from build123d import *

# Parameters (mm, degrees)
SKETCH2_W           = 106
SKETCH2_H           = 106
SKETCH2_R           = 4
SKETCH2_R_2         = 6
BOSS_EXTRUDE1_DEPTH = 25
SKETCH3_W           = 106
SKETCH3_H           = 106
SKETCH3_W_2         = 100
SKETCH3_H_2         = 100
BOSS_EXTRUDE2_DEPTH = 20
SKETCH5_W           = 3
SKETCH5_H           = 23
BOSS_EXTRUDE3_DEPTH = 20
SKETCH7_W           = 20
SKETCH7_H           = 3
BOSS_EXTRUDE4_DEPTH = 20
SKETCH10_W          = 10
SKETCH10_H          = 4
BOSS_EXTRUDE5_DEPTH = 10
SKETCH11_W          = 10
SKETCH11_H          = 4
BOSS_EXTRUDE6_DEPTH = 10
FILLET2_RADIUS      = 5
FILLET2_LENGTH      = 4
FILLET3_R           = 5
FILLET4_R           = 5
FILLET5_R           = 5
SKETCH13_R          = 1.6
CUT_EXTRUDE2_DEPTH  = 163.397660082
SKETCH14_W          = 35.96051594
SKETCH14_H          = 7.693498276
CUT_EXTRUDE3_DEPTH  = 30


with BuildPart() as part:
    # Sketch2 → Boss-Extrude1 (new body)
    with BuildSketch(Plane(origin=(0, 0, 0), x_dir=(1, 0, 0), z_dir=(0, 1, 0))):
        with Locations((53, 53)):
            Rectangle(SKETCH2_W, SKETCH2_H)
        with Locations(Location((18, 15, 0), (0, 0, 270))):
            Circle(SKETCH2_R, mode=Mode.SUBTRACT)
        with Locations(Location((92, 13.5, 0), (0, 0, 270))):
            Circle(SKETCH2_R_2, mode=Mode.SUBTRACT)
    extrude(amount=BOSS_EXTRUDE1_DEPTH)

    # Sketch3 → Boss-Extrude2 (add)
    with BuildSketch(Plane(origin=(0, 25, 0), x_dir=(1, 0, 0), z_dir=(0, 1, 0))):
        with Locations((53, 53)):
            Rectangle(SKETCH3_W, SKETCH3_H)
        with Locations((53, 53)):
            Rectangle(SKETCH3_W_2, SKETCH3_H_2, mode=Mode.SUBTRACT)
    extrude(amount=BOSS_EXTRUDE2_DEPTH)

    # Sketch5 → Boss-Extrude3 (add)
    with BuildSketch(Plane(origin=(0, 25, 0), x_dir=(1, 0, 0), z_dir=(0, 1, 0))):
        Polygon((3, 28), (3, 25), (34, 25), (34, 23), (37, 23), (37, 43), (34, 43), (34, 28), align=None)
        Polygon((83, 52.5), (83, 26.5), (76, 26.5), (76, 3), (73, 3), (73, 29.5), (80, 29.5), (80, 49.5), (73, 49.5), (73, 52.5), align=None)
        Polygon((3, 63), (3, 60), (29, 60), (29, 80), (26, 80), (26, 63), align=None)
        with Locations((57.5, 14.5)):
            Rectangle(SKETCH5_W, SKETCH5_H)
    extrude(amount=BOSS_EXTRUDE3_DEPTH)

    # Sketch7 → Boss-Extrude4 (add)
    with BuildSketch(Plane(origin=(0, 25, 0), x_dir=(1, 0, 0), z_dir=(0, 1, 0))):
        Polygon((50, 67.496539), (53, 67.496539), (53, 70.496539), (53, 79.996539), (50, 79.996539), align=None)
        with Locations((63, 68.996539)):
            Rectangle(SKETCH7_W, SKETCH7_H)
        Polygon((73, 67.496539), (73, 52.5), (76, 52.5), (76, 80), (73, 80), (73, 70.496539), align=None)
    extrude(amount=BOSS_EXTRUDE4_DEPTH)

    # Sketch10 → Boss-Extrude5 (add)
    with BuildSketch(Plane.XY):
        with Locations((53, 2)):
            Rectangle(SKETCH10_W, SKETCH10_H)
    extrude(amount=BOSS_EXTRUDE5_DEPTH)

    # Sketch11 → Boss-Extrude6 (add)
    with BuildSketch(Plane(origin=(0, 0, -106), x_dir=(-1, 0, 0), z_dir=(0, 0, -1))):
        with Locations((-53, 2)):
            Rectangle(SKETCH11_W, SKETCH11_H)
    extrude(amount=BOSS_EXTRUDE6_DEPTH)

    # Fillet2: full round fillet: the end face becomes a half cylinder, R = half its width
    fillet2_face = Plane((53, 2, -116), x_dir=(0, -1, 0), z_dir=(0, 0, -1))  # on the end face: x along it, z out of the body
    fillet2_slab = fillet2_face.offset(-FILLET2_RADIUS / 2) * Box(FILLET2_LENGTH, 2 * FILLET2_RADIUS, FILLET2_RADIUS, mode=Mode.PRIVATE)  # the body's end, R deep
    fillet2_round = Plane((53, 2, -111), x_dir=(0, 0, -1), z_dir=(0, -1, 0)) * Cylinder(FILLET2_RADIUS, FILLET2_LENGTH, mode=Mode.PRIVATE)  # its axis R under the face
    add(fillet2_slab - fillet2_round, mode=Mode.SUBTRACT)

    # Fillet3
    fillet3_edges = [part.edges().sort_by_distance(p)[0] for p in [
        (48, 2, -106),
        (58, 2, -106),
    ]]
    fillet(fillet3_edges, radius=FILLET3_R - 0.0001)  # a hair under: the kernel refuses the full size

    # Fillet4
    fillet4_edges = [part.edges().sort_by_distance(p)[0] for p in [
        (48, 2, 0),
        (58, 2, 0),
    ]]
    fillet(fillet4_edges, radius=FILLET4_R)

    # Fillet5
    fillet5_edges = [part.edges().sort_by_distance(p)[0] for p in [
        (48, 2, 10),
        (58, 2, 10),
    ]]
    fillet(fillet5_edges, radius=FILLET5_R - 0.0001)  # a hair under: the kernel refuses the full size

    # Sketch13 → Cut-Extrude2 (cut, through all)
    with BuildSketch(Plane(origin=(0, 4, 0), x_dir=(1, 0, 0), z_dir=(0, 1, 0))):
        with Locations(Location((53, -5, 0), (0, 0, 180))):
            Circle(SKETCH13_R)
        with Locations(Location((53, 111, 0), (0, 0, 180))):
            Circle(SKETCH13_R)
    extrude(amount=-CUT_EXTRUDE2_DEPTH, mode=Mode.SUBTRACT)

    # Sketch14 → Cut-Extrude3 (cut)
    with BuildSketch(Plane.XY):
        with Locations((88.01974203, 3.846749138)):
            Rectangle(SKETCH14_W, SKETCH14_H)
    extrude(amount=-CUT_EXTRUDE3_DEPTH, mode=Mode.SUBTRACT)


solid = part.part
Here's how the part is built. I have some questions about the finished solid (model axes, mm). A direction names the side the tool comes from. Coordinates: 2 decimals unless noted, no trailing zeros. Write each loop counter-clockwise with the first axis right and the second up, starting at its lowest first coordinate (ties: lowest second). Pieces come first, ordered by that corner, then holes. Notation, with made-up numbers: (37, 2.5) - (90, 2.5) arc R9 cw to (90, 13.5) - close; hole circle Ø10 at (62.5, -19). An arc over 180 degrees is marked (long way). Use one line per item in the form item = value.
1) Suppose I cut it at A-A, the plane x = 18. Write out the boundary of the cut face in (y, z).
Solved:
outline = (0, -106) - (45, -106) - (45, -103) - (25, -103) - (25, -63) - (45, -63) - (45, -60) - (25, -60) - (25, -28) - (45, -28) - (45, -25) - (25, -25) - (25, -19) - (0, -19) - close; (0, -11) - (25, -11) - (25, -3) - (45, -3) - (45, 0) - (0, 0) - close
2) Suppose I cut it at B-B, the plane z = -88. Write out the boundary of the cut face in (x, y).
Solved:
outline = (0, 0) - (106, 0) - (106, 45) - (103, 45) - (103, 25) - (3, 25) - (3, 45) - (0, 45) - close
3) Suppose I cut it at C-C, the plane z = -15. Write out the boundary of the cut face in (x, y).
Solved:
outline = (0, 0) - (14, 0) - (14, 25) - (3, 25) - (3, 45) - (0, 45) - close; (22, 0) - (70.04, 0) - (70.04, 7.69) - (86.19, 7.69) - (86.19, 25) - (76, 25) - (76, 45) - (73, 45) - (73, 25) - (59, 25) - (59, 45) - (56, 45) - (56, 25) - (22, 25) - close; (97.81, 7.69) - (106, 7.69) - (106, 45) - (103, 45) - (103, 25) - (97.81, 25) - close
4) Suppose I cut it at D-D, the plane z = -36. Write out the boundary of the cut face in (x, y).
Solved:
outline = (0, 0) - (106, 0) - (106, 45) - (103, 45) - (103, 25) - (83, 25) - (83, 45) - (80, 45) - (80, 25) - (37, 25) - (37, 45) - (34, 45) - (34, 25) - (3, 25) - (3, 45) - (0, 45) - close
5) On a 3-axis mill with a long thin cutter (end or side, diameter ignored), from which of +Z, -Z, +X, -X, +Y, -Y can I reach the whole of each face in a straight line? I mean faces 5 (the cylindrical face through (97.059, 16.226, -10.274)), 6 (the flat face through (73, 35, -59)), 7 (the flat face through (87.8, 7.693, -18.1)). Say none if no direction works.
Solved:
face_5 = +Y, -Y
face_6 = +Y
face_7 = +Z, +X, -Y
6) I'm going to push flat-ended pins straight in: P1, Ø8, axis at x = 65.5, z = -40.5, coming from the +Y side; P2, Ø2.5, axis at y = 2.5, z = -10, coming from the +X side; P3, Ø16, axis at x = 60, y = 35, coming from the +Z side. Where does each tip first touch, or does it pass through?
Solved:
P1 = 25
P2 = 70.04
P3 = 0
7) Thinking about a two-plate mould opening in X: for faces 1 (the flat face through (70.039, 4, -15)), 2 (the cylindrical face through (49, 2, 8)), 3 (the flat face through (53, 4, 3)), 4 (the flat face through (52, 35, -103)), which applies, released by +X, released by -X, zero draft, split by the parting line, or undercut?
Solved:
face_1 = released by +X
face_2 = released by -X
face_3 = zero draft
face_4 = undercut
8) I need wall thicknesses on line 1 (X direction, y = 33.5, z = -48); line 2 (Z direction, x = 14, y = 34); line 3 (X direction, y = 36.5, z = -21.5). Which ranges of each line are inside material? Lowest first, please.
Solved:
line_1 = 0 to 3, 80 to 83, 103 to 106
line_2 = -106 to -103, -63 to -60, -28 to -25, -3 to 0
line_3 = 0 to 3, 56 to 59, 73 to 76, 103 to 106
